Geometry check sheet. Reference: the model listing, model coordinates, mm. A direction names the side the tool comes from. Round coordinates to 2 decimals unless told otherwise and drop trailing zeros. Order: outer loops, then holes, each group sorted by start corner. A loop starts at its lowest first (then second) coordinate and runs counter-clockwise, first axis right, second up.
(1) Set-up check for faces 4 (the face through (11.923, 3.755, 249.352)), 5 (the face through (5.77, -11.09, 413.25)), 6 (the face through (-4, 7, 309)): record each of +Z, -Z, +X, -X, +Y, -Y from which the full face is reachable in a straight line by a thin tool's end or side.
(2) Go/stop test with flat-tipped pins: pin 1 (4.5 mm diameter, centred on y = 8, z = 166.5, fed in from -X); pin 2 (9 mm diameter, centred on x = 0.5, z = 171, fed in from +Y); pin 3 (5 mm diameter, centred on x = -9.5, z = 66.5, fed in from +Y). Record where each tip stops, or that it passes through.
(3) Material ranges on line 1 along Z through (x, y) = (-3, 4.5) (3 decimals); line 2 along Z through (x, y) = (-7.5, -12) (3 decimals); line 3 along X through (y, z) = (-10.5, 39), recorded low to high.
(4) Release check for a two-part mould opening along X. For faces 1 (the face through (4, 7, 309)), 2 (the face through (5.77, -11.09, 103.17)), 3 (the face through (4.3, -12.1, 229.275)) record: +X half, -X half, draft (parallel to the pull), parting line (faces both ways), or undercut.
(5) Sectioned sample at A-A (z = 485.5). Record the boundary of the cut face in (x, y), plus the area to 3 significant figures.
from build123d import *

# Parameters (mm, degrees)
SKETCH1_R           = 12.5
BOSS_EXTRUDE1_DEPTH = 500
SKETCH6_R           = 12.5
BOSS_EXTRUDE2_DEPTH = 40
CUT_EXTRUDE1_DEPTH  = 10
SKETCH8_W           = 8
SKETCH8_H           = 37
CUT_EXTRUDE2_DEPTH  = 10


with BuildPart() as part:
    # Sketch1 → Boss-Extrude1 (new body)
    with BuildSketch(Plane.XY):
        Circle(SKETCH1_R)
    extrude(amount=BOSS_EXTRUDE1_DEPTH)

    # Loft1: read off the stored shape, not the designer's step
    # Loft1: loft between two sections, ruled curve by curve
    loft1_from = [
        Edge.make_bspline([(12.212340856, -8.709691775, 229.275), (-5.207042693, -33.134373487, 229.275), (-29.631724406, -15.714989938, 229.275), (-12.212340856, 8.709691775, 229.275), (5.207042693, 33.134373487, 229.275), (29.631724406, 15.714989938, 229.275), (12.212340856, -8.709691775, 229.275)], [0, 0, 0, 0, 0.5, 0.5, 0.5, 1, 1, 1, 1], 3, [1, 0.333333333, 0.333333333, 1, 0.333333333, 0.333333333, 1]),
    ]
    loft1_to = [
        Edge.make_bspline([(11.08117333, -12.89215256, 209.275), (-14.70313179, -35.05449922, 209.275), (-36.86547845, -9.2701941, 209.275), (-11.08117333, 12.89215256, 209.275), (14.70313179, 35.05449922, 209.275), (36.86547845, 9.2701941, 209.275), (11.08117333, -12.89215256, 209.275)], [0, 0, 0, 0, 0.5, 0.5, 0.5, 1, 1, 1, 1], 3, [1, 0.333333333, 0.333333333, 1, 0.333333333, 0.333333333, 1]),
    ]
    loft1 = Solid(Shell([*[Face.make_surface_from_curves(loft1_from[k], loft1_to[k]) for k in range(1)], Face(Wire(loft1_from)), Face(Wire(loft1_to))]))
    add(loft1)

    # Loft2: read off the stored shape, not the designer's step
    # Loft2: loft between two sections, ruled curve by curve
    loft2_from = [
        Edge.make_bspline([(-16.92047911, -1.642372271, 290), (-20.205223652, 32.19858595, 290), (13.635734568, 35.483330492, 290), (16.92047911, 1.642372271, 290), (20.205223652, -32.19858595, 290), (-13.635734568, -35.483330492, 290), (-16.92047911, -1.642372271, 290)], [0, 0, 0, 0, 0.5, 0.5, 0.5, 1, 1, 1, 1], 3, [1, 0.333333333, 0.333333333, 1, 0.333333333, 0.333333333, 1]),
    ]
    loft2_to = [
        Edge.make_bspline([(-12.135254916, 8.816778784, 270), (5.498302653, 33.087288616, 270), (29.768812484, 15.453731047, 270), (12.135254916, -8.816778784, 270), (-5.498302653, -33.087288616, 270), (-29.768812484, -15.453731047, 270), (-12.135254916, 8.816778784, 270)], [0, 0, 0, 0, 0.5, 0.5, 0.5, 1, 1, 1, 1], 3, [1, 0.333333333, 0.333333333, 1, 0.333333333, 0.333333333, 1]),
    ]
    loft2 = Solid(Shell([*[Face.make_surface_from_curves(loft2_from[k], loft2_to[k]) for k in range(1)], Face(Wire(loft2_from)), Face(Wire(loft2_to))]))
    add(loft2)

    # Sketch6 → Boss-Extrude2 (add)
    with BuildSketch(Plane.XY.offset(500)):
        Circle(SKETCH6_R)
    extrude(amount=BOSS_EXTRUDE2_DEPTH)

    # Sketch9 → Cut-Extrude1 (cut)
    with BuildSketch(Plane(origin=(0, 12.5, 0), x_dir=(1, 0, 0), z_dir=(0, 1, 0))):
        Polygon((-4, -146.275), (-4, -209.275), (0, -209.275), (4, -209.275), (4, -146.275), align=None)
    extrude(amount=-CUT_EXTRUDE1_DEPTH, mode=Mode.SUBTRACT)

    # Sketch8 → Cut-Extrude2 (cut)
    with BuildSketch(Plane(origin=(0, 12.5, 0), x_dir=(1, 0, 0), z_dir=(0, 1, 0))):
        with Locations((0, -308.5)):
            Rectangle(SKETCH8_W, SKETCH8_H)
    extrude(amount=-CUT_EXTRUDE2_DEPTH, mode=Mode.SUBTRACT)


solid = part.part
Answer below:
1. face 4: none
1. face 5: +Z
1. face 6: +Y
2. pin 1: stops at x = -11.1
2. pin 2: stops at y = 11.84
2. pin 3: stops at y = 10.36
3. line 1: z = 0 to 146.275, 209.275 to 290, 327 to 540
3. line 2: z = 209.275 to 229.275, 270 to 290
3. line 3: x = -6.78 to 6.78
4. face 1: undercut
4. face 2: parting line
4. face 3: draft
5. outline: circle Ø25 at (0, 0)
5. area: 491 mm2
